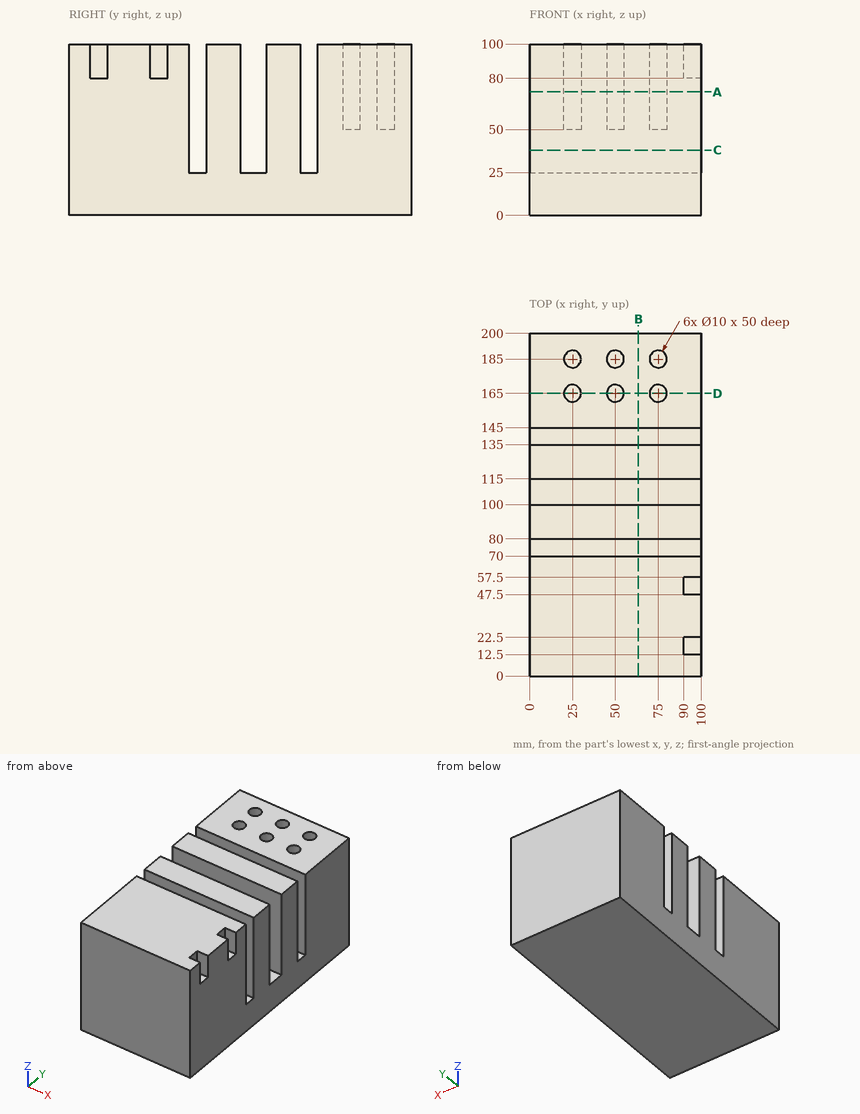
Could you check a few things on this drawing? It's one solid part, dimensions in mm from its lowest x, y, z. Give positions to 0.01 mm unless a question says otherwise; leave off trailing zeros. Order: outer loops, then holes, each group sorted by start corner. A loop starts at its lowest first (then second) coordinate and runs counter-clockwise, first axis right, second up. Notation, with made-up numbers: (-11.5, 87.5) -> (35.5, 87.5) arc R19 ccw to (35.5, 106.5) -> close; hole circle Ø6 at (75.5, 83.25). An arc over 180 degrees is marked (long way). Answer in a Markdown table with one row per item. Add a question column.
Item 1: Imagine slicing it at C-C (z = 38). List the corners of the cut face in (x, y) for me, and give its area (3 significant figures).
Item 2: Please list where these lines run through material, in increasing order: probe 1 along Y at (x, z) = (24.5, 33); probe 2 along Y at (x, z) = (25, 79); probe 3 along Z at (x, y) = (51, 189).
Item 3: Imagine slicing it at A-A (z = 72). Count the separate pieces of the cut face and the enclosed holes in it, and give its area (3 significant figures).
Item 4: I'm going to push flat-ended pins straight in: P1, Ø6, axis at x = 88, y = 32, coming from the -Z side; P2, Ø5, axis at x = 23, y = 184.5, coming from the +Z side; P3, Ø8, axis at y = 52.5, z = 90.5, coming from the +X side; P4, Ø4.5, axis at x = 46.5, y = 104, coming from the +Z side. Where does each tip first touch, or does it pass through?
Item 5: Imagine slicing it at B-B (x = 63.5). List the corners of the cut face in (y, z) for me.
Item 6: Imagine slicing it at D-D (y = 165). List the corners of the cut face in (x, z) for me.
Result:
| question | item | result |
|---|---|---|
| 1 | outline | (0, 0) -> (100, 0) -> (100, 70) -> (0, 70) -> close; (0, 80) -> (100, 80) -> (100, 100) -> (0, 100) -> close; (0, 115) -> (100, 115) -> (100, 135) -> (0, 135) -> close; (0, 145) -> (100, 145) -> (100, 200) -> (0, 200) -> close |
| 1 | area | 16,500 mm2 |
| 2 | probe 1 | 0 to 70, 80 to 100, 115 to 135, 145 to 200 |
| 2 | probe 2 | 0 to 70, 80 to 100, 115 to 135, 145 to 160, 170 to 180, 190 to 200 |
| 2 | probe 3 | 0 to 50 |
| 3 | separate pieces | 4 |
| 3 | enclosed holes | 6 |
| 3 | area | 16,000 mm2 |
| 4 | P1 | z = 0 |
| 4 | P2 | z = 50 |
| 4 | P3 | x = 90 |
| 4 | P4 | z = 25 |
| 5 | outline | (0, 0) -> (200, 0) -> (200, 100) -> (145, 100) -> (145, 25) -> (135, 25) -> (135, 100) -> (115, 100) -> (115, 25) -> (100, 25) -> (100, 100) -> (80, 100) -> (80, 25) -> (70, 25) -> (70, 100) -> (0, 100) -> close |
| 6 | outline | (0, 0) -> (100, 0) -> (100, 100) -> (80, 100) -> (80, 50) -> (70, 50) -> (70, 100) -> (55, 100) -> (55, 50) -> (45, 50) -> (45, 100) -> (30, 100) -> (30, 50) -> (20, 50) -> (20, 100) -> (0, 100) -> close |
